Build history of the part. All positions in model axes, mm. A direction names the side the tool comes from. Round coordinates to 2 decimals unless told otherwise and drop trailing zeros. Write each loop counter-clockwise with the first axis right and the second up, starting at its lowest first coordinate (ties: lowest second). Pieces come first, ordered by that corner, then holes. Notation, with made-up numbers: M -22,-25 L 29,-25 A16 cw 29,-1 Z; hole C 57.25,69.5 d8. An arc over 180 degrees is marked long. Write item = value, one per line. Start each with the question number.
Q1. Drop flat-ended pins along their axis: P1, Ø10.5, axis at y = -24, z = 6, coming from the +X side; P2, Ø9, axis at x = 17.5, z = 0, coming from the +Y side; P3, Ø1, axis at x = 14.5, z = 10.5, coming from the -Y side; P4, Ø1.5, axis at x = 92.5, z = -1.5, coming from the +Y side. Give the stop position or say it passes through.
Q2. Band-saw the part on C-C on y = -15. Write the cut outline in (x, z), plus the area to 4 significant figures.
Q3. Pull direction X, two halves, no side cores. Call faces 1 (the cylindrical face through (97.437, -58.713, -4.216)), 2 (the flat face through (71, -8, -17.5)), 3 (the cylindrical face through (80.805, -54.313, -0.245)): released by +X, released by -X, zero draft, split by the parting line, or undercut.
Q4. Tool access for faces 4 (the flat face through (87.5, -23, 0)), 5 (the flat face through (38, -10, 0)), 6 (the cylindrical face through (4.99, -5.07, -12.24)): list every direction of +Z, -Z, +X, -X, +Y, -Y with a clear straight run to the whole face (end or side of a thin tool).
Q5. Probe L1, parallel to Z at x = 17.5, y = -3.25; L2, parallel to Y at x = 61, z = 14.5; L3, parallel to X at y = -42, z = -3.5. List the from-to ranges inside material, lowest first.
Q6. Band-saw the part on A-A on y = -30. Write the cut outline in (x, z), plus the area to 4 significant figures.
Q7. Band-saw the part on B-B on x = 27. Write the cut outline in (y, z).
Autodesk Inventor part; units mm, degrees
ref_plane "YZ Plane" through (0, 0, 0) normal (1, 0, 0) x (0, 1, 0)
ref_plane "XZ Plane" through (0, 0, 0) normal (0, 1, 0) x (-1, 0, 0)
ref_plane "XY Plane" through (0, 0, 0) normal (0, 0, 1) x (1, 0, 0)
sketch "스케치1" plane through (0, 0, 0) normal (0, 0, 1) x (1, 0, 0)
  line L0 (0, 0) -> (0, -10)
  line L1 (0, -10) -> (80, -10)
  line L2 (80, -10) -> (80, -54.778)
  line L3 (80, -54.778) -> (102.4565, -65.2497)
  line L4 (102.4565, -65.2497) -> (105.6262, -58.4524)
  line L5 (105.6262, -58.4524) -> (87.5, -50)
  line L6 (87.5, -50) -> (87.5, 0)
  line L7 (87.5, 0) -> (0, 0)
  dimension "d5" = 7.5
  dimension "d7" = 20
  dimension "d9" = 7.5
  dimension "d10" = 50
  dimension "d11" = 10
  dimension "d12" = 115
  dimension "d13" = 87.5
extrude "돌출1" add sketch "스케치1" along normal mid plane 35
fillet "모깎기1" radius 17.5 1 edges at (0, -5, -17.5)
fillet "모깎기2" radius 17.5 1 edges at (0, -5, 17.5)
fillet "모깎기3" radius 2 1 edges at (80, -10, 0)
fillet "모깎기5" radius 5 1 edges at (80, -54.778, 0)
sketch "스케치3" plane through (87.5, 0, 17.5) normal (0, 1, 0) x (1, 0, 0)
  arc A0 (-70, 35) -> (-70, 0) centre (-70, 17.5) ccw
  circle A1 centre (-70, 17.5) radius 7.5
  point P0 (-87.5, 17.5)
  dimension "d22" = 15
sketch "스케치4" plane through (87.5, -50, 17.5) normal (0.4226183, 0.9063078, 0) x (0.9063078, -0.4226183, 0)
  circle A0 centre (10, 17.5) radius 5
  line L0 (0, 35) -> (0, 0)
  point P0 (-100.4328, 17.5)
  dimension "d23" = 10
  dimension "d24" = 10
ref_plane "작업 평면1" through (0, 0, 0) normal (0, 0, 1) x (1, 0, 0)
fillet "모깎기7" radius 5 1 edges at (87.5, 0, 0)
sketch "스케치6" plane through (0, 0, 0) normal (0, 0, 1) x (1, 0, 0)
  line L0 (37.61, 21.4494) -> (161.1108, -36.1399)
  arc A0 (87.5, -5) -> (82.5, 0) centre (82.5, -5) ccw
  line L1 (17.5, 0) -> (82.5, 0)
  point P0 (0, 0)
  dimension "d26" = 25
ref_plane "작업 평면2" through (161.1108, -36.1399, 0) normal (0.9063078, -0.4226183, 0) x (0.4226183, 0.9063078, 0)
sketch "스케치7" plane through (161.1108, -36.1399, 0) normal (0.9063078, -0.4226183, 0) x (0.4226183, 0.9063078, 0)
  point P0 (-35.3345, 0)
sketch "스케치8" plane through (161.1108, -36.1399, 0) normal (0.9063078, -0.4226183, 0) x (0.4226183, 0.9063078, 0)
  point P0 (-35.3345, 0)
sketch "스케치9" plane through (161.1108, -36.1399, 0) normal (0.9063078, -0.4226183, 0) x (0.4226183, 0.9063078, 0)
  line L0 (0, -17.5) -> (0, 17.5)
  circle A0 centre (0, 0) radius 7
  point P0 (-35.3345, 0)
  dimension "d27" = 14
extrude "돌출2" cut sketch "스케치9" against normal blind 200
extrude "돌출3" cut sketch "스케치3" against normal blind 200
extrude "돌출4" cut sketch "스케치4" against normal blind 200
sketch "스케치10" plane through (87.5, -50, 17.5) normal (1, 0, 0) x (0, 0, -1)
  circle A0 centre (17.5, 20) radius 5
  line L0 (10.5157, 50) -> (24.4843, 50)
  point P0 (17.5, 50)
  dimension "d34" = 10
  dimension "d35" = 30
extrude "돌출5" cut sketch "스케치10" against normal blind 60
properties part number "3번"
Conclusion:
q1.P1 = 87.5
q1.P2 = through
q1.P3 = -10
q1.P4 = -51.98
q2.outline = M 80,-17.5 L 87.5,-17.5 L 87.5,17.5 L 80,17.5 Z
q2.area = 262.5 mm^2
q3.face_1 = undercut
q3.face_2 = zero draft
q3.face_3 = released by -X
q4.face_4 = +Z, -Z, +X, +Y
q4.face_5 = +Z, -Z, -X, -Y
q4.face_6 = -Z, -X, +Y, -Y
q5.L1 = -17.5 to -7.5, 7.5 to 17.5
q5.L2 = -10 to 0
q5.L3 = 80 to 87.5
q6.outline = M 80,-17.5 L 87.5,-17.5 L 87.5,-5 L 80,-5 Z; M 80,5 L 87.5,5 L 87.5,17.5 L 80,17.5 Z
q6.area = 187.5 mm^2
q7.outline = M -10,-17.5 L 0,-17.5 L 0,17.5 L -10,17.5 Z
